from build123d import *

# Parameters (mm, degrees)
F0_W     = 99.3330795318
F0_H     = 54.4778928161
F1_DEPTH = 34.29
F2_R     = 10.414
F3_R     = 6.4262
F4_T     = -2.54
F6_D     = 6.35


with BuildPart() as f1:
    # F0 (on Front) → F1 (new body)
    with BuildSketch(Plane.XZ):
        with Locations((22.2479021177, 0.9583178908)):
            Rectangle(F0_W, F0_H)
    extrude(amount=F1_DEPTH)

    # F2
    f2_edges = [f1.edges().sort_by_distance(p)[0] for p in [
        (71.914442, -17.145, 28.197264),
        (-27.418638, -17.145, 28.197264),
        (71.914442, -34.29, 0.958318),
        (-27.418638, -34.29, 0.958318),
    ]]
    fillet(f2_edges, radius=F2_R)

    # F3
    f3_edges = [f1.edges().sort_by_distance(p)[0] for p in [
        (22.247902, 0, -26.280629),
    ]]
    fillet(f3_edges, radius=F3_R)

    # F4
    f4_openings = [f1.faces().sort_by_distance(p)[0] for p in [
        (22.247902, -34.29, 0.958318),
        (22.247902, -17.145, 28.197264),
        (68.864252, -17.145, 25.147074),
        (68.864252, -31.23981, 0.958318),
        (71.914442, -12.027221, -4.073711),
        (-24.368448, -31.23981, 0.958318),
        (-24.368448, -17.145, 25.147074),
        (-27.418638, -12.027221, -4.073711),
    ]]
    offset(amount=F4_T, openings=f4_openings)

    # F6 (through all)
    with Locations(Plane.XZ.offset(2.54)):
        with Locations((-17.0046376482, 17.7832642988), (61.5004418836, 17.7832642988)):
            Hole(F6_D / 2)


solid = f1.part
Could you check a few things on this model? Use its own coordinates, in mm. A direction names the side the tool comes from. Round coordinates to 2 decimals unless told otherwise and drop trailing zeros. Write each loop counter-clockwise with the first axis right and the second up, starting at its lowest first coordinate (ties: lowest second). Pieces come first, ordered by that corner, then holes. Notation, with made-up numbers: (27, 24.25) - (40, 24.25) arc R32 cw to (40, 61.25) - close; hole circle Ø6 at (-1, 69.25). An arc over 180 degrees is marked (long way). Put each result on its own line as item: value. Start each with the question number.
(1) I need wall thicknesses on probe 1 along Z at (x, y) = (54, -30); probe 2 along Y at (x, z) = (42.5, -0.5); probe 3 along Z at (x, y) = (63, -5.5). Which ranges of each line are inside material? Lowest first, please.
(2) I want a section at C-C, the plane z = -5.5. Please give me the cut outline in (x, y).
(3) I want a section at B-B, the plane y = -21.5. Please give me the cut outline in (x, z), plus the area to 3 significant figures.
(4) I want a section at A-A, the plane x = 52.5. Please give me the cut outline in (y, z).
(5) Will these pins go through, and if not, where does the flat tip stop? pin 1 (24 mm diameter, centred on x = 41.5, z = -4.5, fed in from -Y); pin 2 (8 mm diameter, centred on x = -13.5, y = -17, fed in from +Z); pin 3 (4 mm diameter, centred on y = -4.5, z = 6.5, fed in from +X).
(6) For faces 1 (the flat face through (71.914, -2, -11)), 2 (the flat face through (22, -20, -23.741)), which set-ups out of +Z, -Z, +X, -X, +Y, -Y let a thin tool reach every point of the face, with its end or its side?
(7) Thinking about a two-plate mould opening in Z: for faces 3 (the cylindrical face through (-19.94, -1.25, 16.57)), 4 (the cylindrical face through (-24.449, -1.288, 25.066)), 5 (the flat face through (22, -34.29, -25)), 6 (the cylindrical face through (64.02, -1.25, 15.85)), which applies, released by +Z, released by -Z, zero draft, split by the parting line, or undercut?
Here are the results:
1. probe 1: z = -26.28 to -23.74
1. probe 2: y = -2.54 to 0
1. probe 3: z = -26.21 to -23.63
2. outline: (-27.42, -2.54) - (71.91, -2.54) - (71.91, 0) - (-27.42, 0) - close
3. outline: (-27.42, -26.28) - (71.91, -26.28) - (71.91, -23.74) - (-27.42, -23.74) - close
3. area: 252 mm^2
4. outline: (-34.29, -26.28) - (-6.43, -26.28) arc R6.43 ccw to (0, -19.85) - (0, 28.2) - (-2.54, 28.2) - (-2.54, -19.85) arc R3.89 cw to (-6.43, -23.74) - (-34.29, -23.74) - close
5. pin 1: stops at y = -2.54
5. pin 2: stops at z = -23.74
5. pin 3: stops at x = 71.91
6. face 1: +Z, -Z, +X, +Y, -Y
6. face 2: +Z, +X, -X, -Y
7. face 3: undercut
7. face 4: released by +Z
7. face 5: zero draft
7. face 6: undercut
